```python
from build123d import *

# Parameters (mm, degrees)
F1_DEPTH = 60
F2_W     = 5.437252
F2_H     = 3.403648
F2_W_2   = 4.52817
F2_H_2   = 4.068502
F3_DEPTH = 6.3
F2_H_3   = 4.993211
F4_DEPTH = 4.2
F2_H_4   = 4.021845
F5_DEPTH = 5
F2_W_3   = 4.367254
F2_H_5   = 4.921976
F6_DEPTH = 4.6
F2_H_6   = 3.894821
F7_DEPTH = 4.6


with BuildPart() as f1:
    # F0 (on Top) → F1 (new body, symmetric)
    with BuildSketch(Plane.XY):
        Polygon((-9.043264, 0), (-9.043264, 7), (-16.043264, 7), (-16.043264, 0), (-16.043264, -7.59036), (-9.043264, -7.59036), align=None)
    extrude(amount=F1_DEPTH, both=True)

    # F2 (on face) → F3 (join)
    with BuildSketch(Plane.YZ.offset(-9.043264)):
        with Locations((0, 49.416557)):
            Rectangle(F2_W, F2_H)
        with Locations((0, -49.225945)):
            Rectangle(F2_W_2, F2_H_2)
    extrude(amount=F3_DEPTH)

    # F2 (on face) → F4 (join)
    with BuildSketch(Plane.YZ.offset(-9.043264)):
        with Locations((0, 19.678933)):
            Rectangle(F2_W, F2_H_3)
    extrude(amount=F4_DEPTH)

    # F2 (on face) → F5 (join)
    with BuildSketch(Plane.YZ.offset(-9.043264)):
        with Locations((0, 35.789437)):
            Rectangle(F2_W, F2_H_4)
    extrude(amount=F5_DEPTH)

    # F2 (on face) → F6 (join)
    with BuildSketch(Plane.YZ.offset(-9.043264)):
        Rectangle(F2_W_3, F2_H_5)
    extrude(amount=F6_DEPTH)

    # F2 (on face) → F7 (join)
    with BuildSketch(Plane.YZ.offset(-9.043264)):
        with Locations((-2.264085, -23.966038)):
            Rectangle(F2_W_2, F2_H_6)
    extrude(amount=F7_DEPTH)


solid = f1.part
```
Work out the finished part from the listing and answer in its coordinate system (mm). A direction names the side the tool comes from. Give positions to 0.01 mm unless a question says otherwise; leave off trailing zeros. Order: outer loops, then holes, each group sorted by start corner. A loop starts at its lowest first (then second) coordinate and runs counter-clockwise, first axis right, second up. Notation, with made-up numbers: (-24, 68.5) - (29, 68.5) arc R29 ccw to (29, 102.5) - close; hole circle Ø8 at (-3.5, 57). An arc over 180 degrees is marked (long way). One line per item, written item: value. Start each with the question number.
1. Section B-B, the plane y = -6 is taken. Write down the section's boundary in (x, z), then the cut area to 3 significant figures.
2. Which of the six approach directions +Z, -Z, +X, -X, +Y, -Y give full straight-line access (tool end or side, diameter ignored) to faces 1 (the face through (-7, -2.184, 0)), 2 (the face through (-7, -2.719, 36)), 3 (the face through (-7, 2.184, 0)), 4 (the face through (-7, 0, 22.176)), 5 (the face through (-7, 2.719, 20))?
3. Each of these flat-tipped pins is pushed along its axis until it touches: pin 1 Ø1.2 at (x, z) = (-6, 36) entering from +Y; pin 2 Ø4.5 at (x, y) = (-6.5, 0) entering from +Z; pin 3 Ø3.5 at (x, y) = (-6, -1.5) entering from -Z. Where does it stop, or does it pass through?
4. Section A-A, the plane z = 21 is taken. Write down the section's boundary in (x, y).
5. Section C-C, the plane z = -4 is taken. Write down the section's boundary in (x, y).
6. Consider line 1 (Z direction, x = -4.5, y = 1.25); line 2 (Z direction, x = -3.5, y = -0.25); line 3 (X direction, y = 2.5, z = 52). Determine where each line is inside the solid, lowest interval first.
Filled sheet:
1. outline: (-16.04, -60) - (-9.04, -60) - (-9.04, 60) - (-16.04, 60) - close
1. area: 840 mm²
2. face 1: +X, -Y
2. face 2: +Z, +X, -Y
2. face 3: +X, +Y
2. face 4: +X, +Y, -Y
2. face 5: +Z, -Z, +X, +Y
3. pin 1: y = 2.72
3. pin 2: z = 51.12
3. pin 3: z = -51.26
4. outline: (-16.04, -7.59) - (-9.04, -7.59) - (-9.04, -2.72) - (-4.84, -2.72) - (-4.84, 2.72) - (-9.04, 2.72) - (-9.04, 7) - (-16.04, 7) - close
5. outline: (-16.04, -7.59) - (-9.04, -7.59) - (-9.04, 7) - (-16.04, 7) - close
6. line 1: -51.26 to -47.19, -2.46 to 2.46, 33.78 to 37.8, 47.71 to 51.12
6. line 2: -51.26 to -47.19, 47.71 to 51.12
6. line 3: -16.04 to -9.04
